```python
from build123d import *

# Parameters (mm, degrees)
F0_W     = 63.5
F0_H     = 63.5
F1_DEPTH = 12.7
F2_W     = 63.5
F2_H     = 63.5
F3_DEPTH = 12.7
F4_W     = 63.5
F4_H     = 12.7
F5_DEPTH = 50.8
F6_W     = 12.7
F6_H     = 12.7
F7_DEPTH = 50.8
F8_W     = 50.8
F8_H     = 12.7
F9_DEPTH = 63.5


with BuildPart() as f1:
    # F0 (on Front) → F1 (new body)
    with BuildSketch(Plane.XZ):
        with Locations((31.75, -31.75)):
            Rectangle(F0_W, F0_H)
    extrude(amount=F1_DEPTH)

    # F2 (on Right) → F3 (join)
    with BuildSketch(Plane.YZ):
        with Locations((-31.75, -31.75)):
            Rectangle(F2_W, F2_H)
    extrude(amount=F3_DEPTH)

    # F4 (on Front) → F5 (join)
    with BuildSketch(Plane.XZ):
        with Locations((31.75, -57.149136)):
            Rectangle(F4_W, F4_H)
    extrude(amount=F5_DEPTH)

    # F6 (on Right) → F7 (join)
    with BuildSketch(Plane.YZ):
        with Locations((-57.11578, -57.112239)):
            Rectangle(F6_W, F6_H)
    extrude(amount=F7_DEPTH)

    # F8 (on Front) → F9 (join)
    with BuildSketch(Plane.XZ):
        with Locations((25.4, -57.358216)):
            Rectangle(F8_W, F8_H)
    extrude(amount=F9_DEPTH)


solid = f1.part
```
Can you work these out from the model? Positions are in its coordinate system, mm. A direction names the side the tool comes from. Give positions to 0.01 mm unless a question says otherwise; leave off trailing zeros. Loops run counter-clockwise (first coordinate to the right, second up) from the corner with the lowest first, then second, coordinate; pieces in that order, holes last. Notation, with made-up numbers: M -5,-20 L 34,-20 A19 ccw 34,-11 Z; hole C 15,53 d1. An arc over 180 degrees is marked long. Use CSV: the item, a comma, the result in double quotes. Start each with the question number.
1. For P1, Ø1.5, axis at x = 51, y = -18, coming from the +Z side; P2, Ø1.5, axis at x = 30.5, z = -14.5, coming from the +Y side; P3, Ø8, axis at x = 29.5, z = -33.5, coming from the -Y side; P4, Ø10, axis at x = 59, z = -58.5, coming from the -Y side, each with a flat end and sliding along its axis, tell me the tip position at first contact or that it passes through.
2. On a 3-axis mill with a long thin cutter (end or side, diameter ignored), from which of +Z, -Z, +X, -X, +Y, -Y can I reach the whole of each face in a straight line? I mean faces 1 (the face through (10, -18, 0)), 2 (the face through (57, -31, -63.499)), 3 (the face through (57, -50.8, -57)). Say none if no direction works.
3. Imagine slicing it at C-C, the plane z = -20.5. Write out the boundary of the cut face in (x, y).
4. Imagine slicing it at D-D, the plane y = -58.5. Write out the boundary of the cut face in (x, z).
5. If I drill on L1, parallel to X at y = -33, z = -40.5; L2, parallel to Y at x = 41.5, z = -40; L3, parallel to X at y = -60, z = -54, over which ranges is the centre line in solid material (lowest first)?
6. Imagine slicing it at A-A, the plane y = -44. Write out the boundary of the cut face in (x, z), plus the area to 3 significant figures.
Response values:
1,P1,"z = -50.8"
1,P2,"y = 0"
1,P3,"y = -12.7"
1,P4,"y = -50.8"
2,face 1,"+Z, +X, -X, +Y, -Y"
2,face 2,"-Z, +X, +Y, -Y"
2,face 3,"+Z, -Z, +X, -Y"
3,outline,"M 0,-63.5 L 12.7,-63.5 L 12.7,-12.7 L 63.5,-12.7 L 63.5,0 L 0,0 Z"
4,outline,"M 0,-63.71 L 50.8,-63.71 L 50.8,-50.76 L 12.7,-50.76 L 12.7,0 L 0,0 Z"
5,L1,"0 to 12.7"
5,L2,"-12.7 to 0"
5,L3,"0 to 50.8"
6,outline,"M 0,-63.71 L 50.8,-63.71 L 50.8,-63.5 L 63.5,-63.5 L 63.5,-50.8 L 12.7,-50.8 L 12.7,0 L 0,0 Z"
6,area,"1,460 mm^2"
